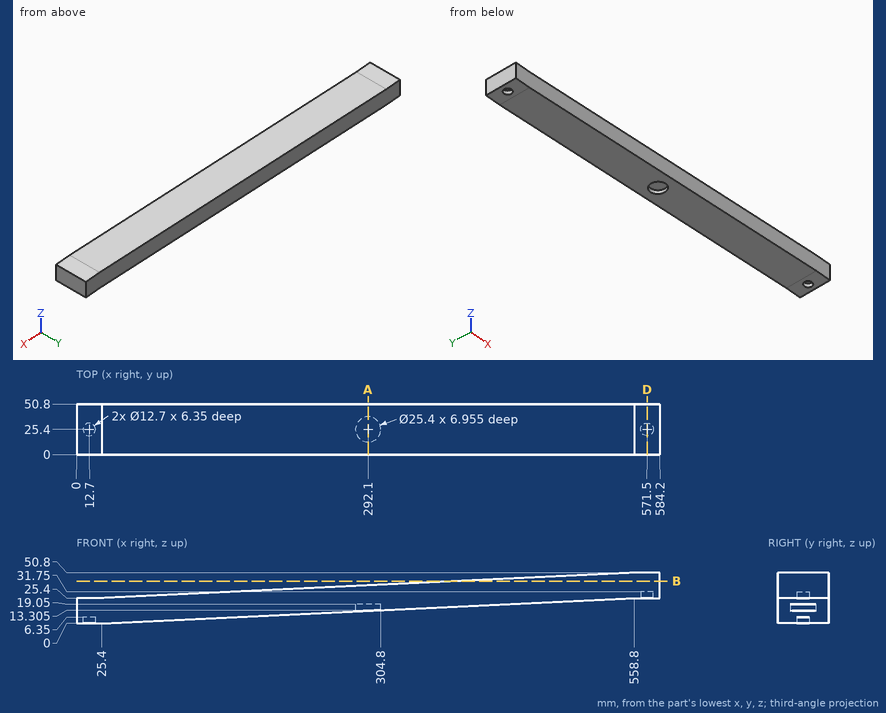
Can you work these out from the drawing? Everything is in mm from the part's minimum corner. Coordinates: 2 decimals unless noted, no trailing zeros. Order: outer loops, then holes, each group sorted by start corner. A loop starts at its lowest first (then second) coordinate and runs counter-clockwise, first axis right, second up. Notation, with made-up numbers: (43, 39) -> (84, 39) arc R18 cw to (84, 68) -> close; hole circle Ø7 at (74.25, 49.25). An arc over 180 degrees is marked (long way). Use one line per item in the form item = value.
Q1. Imagine slicing it at A-A, the plane x = 292.1. List the corners of the cut face in (y, z) for me, then the cut area to 3 significant figures.
From the geometry:
outline = (0, 12.7) -> (12.7, 12.7) -> (12.7, 19.05) -> (38.1, 19.05) -> (38.1, 12.7) -> (50.8, 12.7) -> (50.8, 38.1) -> (0, 38.1) -> close
area = 1,130 mm²
Q2. Will these pins go through, and if not, where does the flat tip stop? P1, Ø2, axis at x = 474.5, y = 24.5, coming from the +Z side; P2, Ø7.5, axis at x = 291.5, y = 27, coming from the -Z side; P3, Ø8, axis at x = 331.5, y = 9.5, coming from the +Z side.
From the geometry:
P1 = 46.83
P2 = 19.05
P3 = 40.17
Q3. I need wall thicknesses on L1, parallel to Y at x = 571, z = 27; L2, parallel to Y at x = 292, z = 14; L3, parallel to Z at x = 305, y = 36. Which ranges of each line are inside material? Lowest first, please.
From the geometry:
L1 = 0 to 19.07, 31.73 to 50.8
L2 = 0 to 12.7, 38.1 to 50.8
L3 = 13.31 to 38.71
Q4. Imagine slicing it at B-B, the plane z = 42.5. List the corners of the cut face in (x, y) for me.
From the geometry:
outline = (384.5, 0) -> (584.2, 0) -> (584.2, 50.8) -> (384.5, 50.8) -> close
Q5. Imagine slicing it at D-D, the plane x = 571.5. List the corners of the cut face in (y, z) for me.
From the geometry:
outline = (0, 25.4) -> (19.05, 25.4) -> (19.05, 31.75) -> (31.75, 31.75) -> (31.75, 25.4) -> (50.8, 25.4) -> (50.8, 50.8) -> (0, 50.8) -> close
